Study the drawing (mm; zero at the part's minimum x, y, z) and answer. Give positions to 0.01 mm unless a question says otherwise; leave off trailing zeros. Write each loop counter-clockwise with the first axis right and the second up, starting at its lowest first coordinate (ties: lowest second). Pieces come first, ordered by that corner, then holes. Notation, with made-up numbers: (10, 9) - (41, 9) arc R15 cw to (41, 38) - close; hole circle Ø10 at (4, 80). An arc over 180 degrees is marked (long way). Answer as CSV lines item,"result".
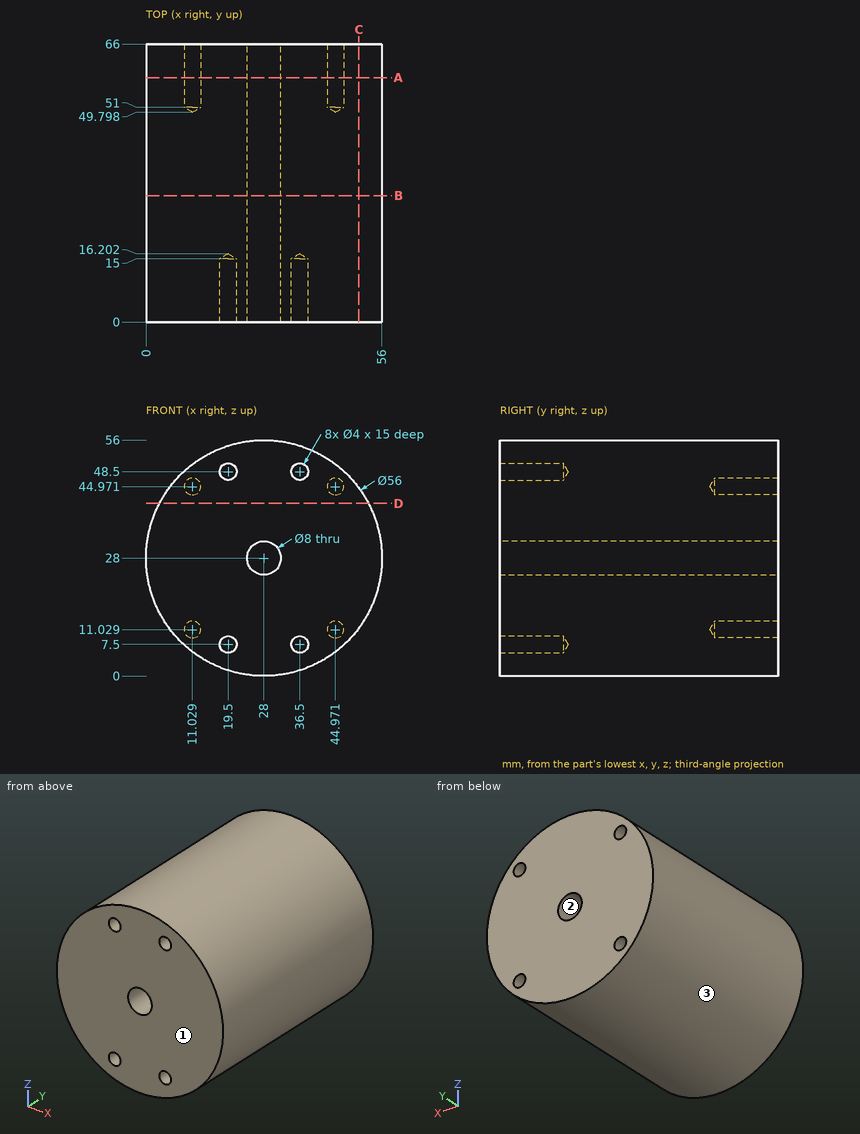
(1) A cutting plane is placed at A-A (y = 58). Write down the section's boundary in (x, z), and give its area (3 significant figures).
Worked out:
outline,"circle Ø56 at (28, 28); hole circle Ø4 at (11.03, 11.03); hole circle Ø4 at (11.03, 44.97); hole circle Ø8 at (28, 28); hole circle Ø4 at (44.97, 11.03); hole circle Ø4 at (44.97, 44.97)"
area,"2,360 mm^2"
(2) Find the intervals of material crossed by L1, parallel to X at y = 19, z = 28; L2, parallel to Z at x = 26, y = 15 (1 decimal); L3, parallel to X at y = 10, z = 7 (1 decimal), in increasing order.
Worked out:
L1,"x = 0 to 24, 32 to 56"
L2,"z = 0.1 to 24.5, 31.5 to 55.9"
L3,"x = 9.5 to 17.6, 21.4 to 34.6, 38.4 to 46.5"
(3) A cutting plane is placed at D-D (z = 41). Write down the section's boundary in (x, y).
Worked out:
outline,"(3.2, 0) - (52.8, 0) - (52.8, 66) - (3.2, 66) - close"
(4) Each of these flat-tipped pins is pushed along its axis until it touches: P1, Ø3, axis at y = 29, z = 46, coming from the +X side; P2, Ø3.5, axis at x = 19.5, z = 48.5, coming from the -Y side; P3, Ø4, axis at y = 14, z = 14.5, coming from the +X side. Where does it stop, or does it pass through?
Worked out:
P1,"stops at x = 50.62"
P2,"stops at y = 15.15"
P3,"stops at x = 53.53"
(5) A cutting plane is placed at C-C (x = 50.5). Write down the section's boundary in (y, z) (1 decimal).
Worked out:
outline,"(0, 11.3) - (66, 11.3) - (66, 44.7) - (0, 44.7) - close"
(6) A cutting plane is placed at B-B (y = 30). Write down the section's boundary in (x, z), and give its area (3 significant figures).
Worked out:
outline,"circle Ø56 at (28, 28); hole circle Ø8 at (28, 28)"
area,"2,410 mm^2"
(7) The mould has two halves that part along Z. Classify the marked faces 1, 2 and 3: +Z half, -Z half, draft (parallel to the pull), parting line (faces both ways), or undercut.
Worked out:
face 1,"draft"
face 2,"undercut"
face 3,"parting line"
